from build123d import *

# Parameters (mm, degrees)
SKETCH_1_R          = 17.5
SKETCH_1_R_2        = 1.75
EXTRUDE_1_DEPTH     = 4
SKETCH_2_R          = 3.2
CUT_EXTRUDE_1_DEPTH = 5
CUT_EXTRUDE_2_DEPTH = 1.9
CHAMFER_1_SIZE      = 1.4


with BuildPart() as part:
    # Эскиз1 → Бобышка-Вытянуть1 (new body)
    with BuildSketch(Plane(origin=(0, 0, 0), x_dir=(1, 0, 0), z_dir=(0, 1, 0))):
        with Locations((0.106470277, -0.341512656)):
            Circle(SKETCH_1_R)
        with Locations((13.106470277, -0.341512656)):
            Circle(SKETCH_1_R_2, mode=Mode.SUBTRACT)
        with Locations((0.106470277, -13.341512656)):
            Circle(SKETCH_1_R_2, mode=Mode.SUBTRACT)
        with Locations((-12.893529723, -0.341512656)):
            Circle(SKETCH_1_R_2, mode=Mode.SUBTRACT)
        with Locations((0.106470277, 12.658487344)):
            Circle(SKETCH_1_R_2, mode=Mode.SUBTRACT)
    extrude(amount=EXTRUDE_1_DEPTH)

    # Эскиз2 → Вырез-Вытянуть1 (cut, through all)
    with BuildSketch(Plane(origin=(0, 4, 0), x_dir=(1, 0, 0), z_dir=(0, 1, 0))):
        with Locations((0.106470277, -0.341512656)):
            Circle(SKETCH_2_R)
    extrude(amount=-CUT_EXTRUDE_1_DEPTH, mode=Mode.SUBTRACT)

    # Эскиз3 → Вырез-Вытянуть2 (cut)
    with BuildSketch(Plane(origin=(0, 4, 0), x_dir=(1, 0, 0), z_dir=(0, 1, 0))):
        with BuildLine():
            Line((6.212000557, 8.808487344), (-5.999060003, 8.808487344))
            ThreePointArc((-5.999060003, 8.808487344), (-7.671704316, 7.436661937), (-9.043529723, 5.764017624))
            Line((-9.043529723, 5.764017624), (-9.043529723, -6.447042936))
            ThreePointArc((-9.043529723, -6.447042936), (-7.671704316, -8.119687249), (-5.999060003, -9.491512656))
            Line((-5.999060003, -9.491512656), (6.212000557, -9.491512656))
            ThreePointArc((6.212000557, -9.491512656), (7.88464487, -8.119687249), (9.256470277, -6.447042936))
            Line((9.256470277, -6.447042936), (9.256470277, 5.764017624))
            ThreePointArc((9.256470277, 5.764017624), (7.88464487, 7.436661937), (6.212000557, 8.808487344))
        make_face()
    extrude(amount=-CUT_EXTRUDE_2_DEPTH, mode=Mode.SUBTRACT)

    # Фаска1
    chamfer_1_edges = [part.edges().sort_by_distance(p)[0] for p in [
        (-14.643529723, 0, 0.341512656),
        (-1.643529723, 0, -12.658487344),
        (11.356470277, 0, 0.341512656),
        (-1.643529723, 0, 13.341512656),
    ]]
    chamfer(chamfer_1_edges, length=CHAMFER_1_SIZE)


solid = part.part
Verification items for the finished model (mm, model axes). A direction names the side the tool comes from. Give positions to 0.01 mm unless a question says otherwise; leave off trailing zeros. Loops run counter-clockwise (first coordinate to the right, second up) from the corner with the lowest first, then second, coordinate; pieces in that order, holes last.
1. Cross-section at D-D on z = -4. Record the cut outline in (x, y), and give its area (3 significant figures).
Derived:
outline: (-16.85, 0) - (17.06, 0) - (17.06, 4) - (9.26, 4) - (9.26, 2.1) - (-9.04, 2.1) - (-9.04, 4) - (-16.85, 4) - close
area: 101 mm2
2. Material ranges on probe 1 along Y at (x, z) = (6, -2.5); probe 2 along Z at (x, y) = (-10.5, 0.35); probe 3 along Z at (x, y) = (12, 0.8), recorded low to high.
Derived:
probe 1: y = 0 to 2.1
probe 2: z = -13.58 to -1.11, 1.79 to 14.26
probe 3: z = -12.5 to -1.73, 2.41 to 13.18
3. Release check for a two-part mould opening along Z. For faces 3 (the flat face through (0, 0, 4)), 4 (the cylindrical face through (7.906, 3.063, -7.415)), 5 (the cylindrical face through (9.514, 1.972, -14.415)), 6 (the flat face through (0, 3, 9.492)) record: +Z half, -Z half, draft (parallel to the pull), parting line (faces both ways), or undercut.
Derived:
face 3: draft
face 4: undercut
face 5: parting line
face 6: undercut
4. Cross-section at C-C on y = 0.75. Record the cut outline in (x, z).
Derived:
outline: circle Ø35 at (0.11, 0.34); hole circle Ø4.8 at (-12.89, 0.34); hole circle Ø6.4 at (0.11, 0.34); hole circle Ø4.8 at (0.11, -12.66); hole circle Ø4.8 at (0.11, 13.34); hole circle Ø4.8 at (13.11, 0.34)
5. Cross-section at A-A on y = 2.75. Record the cut outline in (x, z), and give its area (3 significant figures).
Derived:
outline: circle Ø35 at (0.11, 0.34); hole circle Ø3.5 at (-12.89, 0.34); hole (-9.04, -5.76) arc R11 ccw to (-6, -8.81) - (6.21, -8.81) arc R11 ccw to (9.26, -5.76) - (9.26, 6.45) arc R11 ccw to (6.21, 9.49) - (-6, 9.49) arc R11 ccw to (-9.04, 6.45) - close; hole circle Ø3.5 at (0.11, -12.66); hole circle Ø3.5 at (0.11, 13.34); hole circle Ø3.5 at (13.11, 0.34)
area: 605 mm2
6. Cross-section at B-B on z = -7.5. Record the cut outline in (x, y).
Derived:
outline: (-15.54, 0) - (15.75, 0) - (15.75, 4) - (7.82, 4) - (7.82, 2.1) - (-7.61, 2.1) - (-7.61, 4) - (-15.54, 4) - close
7. Tool access check on faces 1 (the cylindrical face through (-0.121, 2.682, 11.606)), 2 (the cylindrical face through (-7.69, 3.06, 8.1)). Record the directions out of +Z, -Z, +X, -X, +Y, -Y that give a thin tool (end or side, any length) a straight path to the whole face; none if there is none.
Derived:
face 1: +Y, -Y
face 2: +Y
8. Go/stop test with flat-tipped pins: P1, Ø1.5, axis at y = 2.5, z = 1.5, coming from the -X side; P2, Ø1.5, axis at x = 10, y = 1, coming from the +Z side; P3, Ø9, axis at x = 4, z = 1, coming from the +Y side. Record where each tip stops, or that it passes through.
Derived:
P1: stops at x = -17.39
P2: stops at z = 15.26
P3: stops at y = 2.1
